from build123d import *

# Parameters (mm, degrees)
SKETCH006_W     = 266
SKETCH006_H     = 48
PAD003_DEPTH    = 4
SKETCH024_W     = 40
SKETCH024_H     = 30
SKETCH024_W_2   = 30
SKETCH024_H_2   = 20
POCKET007_DEPTH = 4.001
SKETCH031_R     = 12
SKETCH031_R_2   = 1.6
POCKET014_DEPTH = 4.001
SKETCH040_R     = 1.65
HOLE005_DEPTH   = 4.001
SKETCH055_W     = 76
SKETCH055_H     = 10
POCKET021_DEPTH = 4.001


with BuildPart() as part:
    # Sketch006 (on DatumPlane) → Pad003 (new body)
    with BuildSketch(Plane.XZ.offset(-79)):
        with Locations((0, 16)):
            Rectangle(SKETCH006_W, SKETCH006_H)
    extrude(amount=PAD003_DEPTH)

    # Sketch024 (on Face5 of Pad003) → Pocket007 (cut, through all)
    with BuildSketch(Plane(origin=(0, 79, 0), x_dir=(1, 0, 0), z_dir=(0, 1, 0))):
        Polygon((-145, 30), (-100, 30), (-100, 0), (-125, 0), (-125, -15.5), (-155, -15.5), (-155, 4.5), (-145, 4.5), align=None)
        with Locations((-40, 15)):
            Rectangle(SKETCH024_W, SKETCH024_H)
        with Locations((40, 15)):
            Rectangle(SKETCH024_W, SKETCH024_H)
        Polygon((100, 30), (145, 30), (145, 4.5), (155, 4.5), (155, -15.5), (125, -15.5), (125, 0), (100, 0), align=None)
        with Locations((-140, -37.5)):
            Rectangle(SKETCH024_W_2, SKETCH024_H_2)
        with Locations((140, -37.5)):
            Rectangle(SKETCH024_W_2, SKETCH024_H_2)
    extrude(amount=-POCKET007_DEPTH, mode=Mode.SUBTRACT)

    # Sketch031 (on Face2 of Pocket007) → Pocket014 (cut, through all)
    with BuildSketch(Plane(origin=(0, 79, 0), x_dir=(1, 0, 0), z_dir=(0, 1, 0))):
        with Locations((-107, -20.5)):
            Circle(SKETCH031_R)
        with Locations((-116.5, -8.5)):
            Circle(SKETCH031_R_2)
        with Locations((-97.5, -32.5)):
            Circle(SKETCH031_R_2)
        with Locations((-88.5, -8.5)):
            Circle(SKETCH031_R_2)
        with Locations((-79, -20.5)):
            Circle(SKETCH031_R)
        with Locations((-69.5, -32.5)):
            Circle(SKETCH031_R_2)
    extrude(amount=-POCKET014_DEPTH, mode=Mode.SUBTRACT)

    # Sketch040 (on Face2 of Pocket014) → Hole005 (cut, through all)
    with BuildSketch(Plane(origin=(0, 79, 0), x_dir=(1, 0, 0), z_dir=(0, 1, 0))):
        with Locations((39.5, -27)):
            Circle(SKETCH040_R)
    extrude(amount=-HOLE005_DEPTH, mode=Mode.SUBTRACT)

    # Sketch055 (on Face2 of Pocket007) → Pocket021 (cut, through all)
    with BuildSketch(Plane(origin=(0, 79, 0), x_dir=(1, 0, 0), z_dir=(0, 1, 0))):
        with Locations((-91, -41)):
            Rectangle(SKETCH055_W, SKETCH055_H)
    extrude(amount=-POCKET021_DEPTH, mode=Mode.SUBTRACT)


solid = part.part
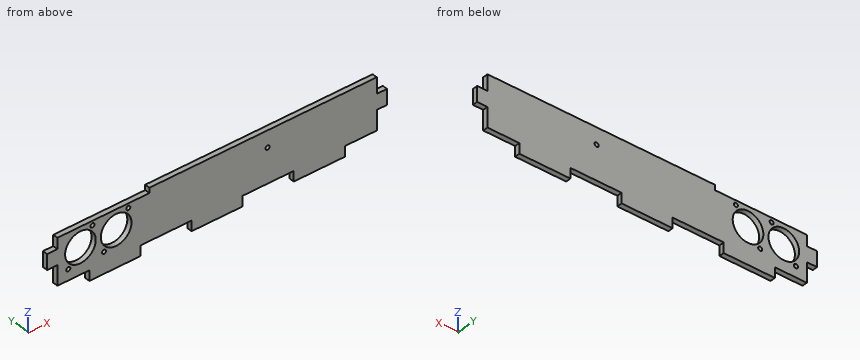
Geometry check sheet. Reference: the model listing, model coordinates, mm. Give positions to 0.01 mm unless a question says otherwise; leave off trailing zeros. Order: outer loops, then holes, each group sorted by start corner. A loop starts at its lowest first (then second) coordinate and runs counter-clockwise, first axis right, second up. Notation, with made-up numbers: (19, 0.5) - (56, 0.5) arc R10 ccw to (56, 4.5) - close; hole circle Ø6 at (-39, -37). An arc over 180 degrees is marked (long way). Answer as a JSON object with one key per item and string values.
(1) Material ranges on line 1 (X direction, y = 77.8, z = -6); line 2 (X direction, y = 76.25, z = 27); line 3 (Z direction, x = -107, y = 77.95), recorded low to high.
Report:
{"line 1": "-100 to -60, -20 to 20, 60 to 100", "line 2": "-133 to -117.09, -96.91 to -89.09, -68.91 to 37.85, 41.15 to 133", "line 3": "0 to 8.5, 32.5 to 36"}
(2) Cross-section at B-B (x = -107). Record the cut outline in (y, z).
Report:
{"outline": "(75, 0) - (79, 0) - (79, 8.5) - (75, 8.5) - close; (75, 32.5) - (79, 32.5) - (79, 36) - (75, 36) - close"}
(3) Depth check by flat-ended pin: pin 1 Ø1.2 at (y, z) = (76.5, -2) entering from +X; pin 2 Ø1.2 at (y, z) = (78, -4.5) entering from -X; pin 3 Ø3.5 at (x, z) = (-88.5, 8.5) entering from +Y; pin 4 Ø1.2 at (x, y) = (38, 76) entering from -Z. Enter the tip coordinate at first touch or a pass-through.
Report:
{"pin 1": "x = 100", "pin 2": "x = -100", "pin 3": "y = 79", "pin 4": "z = 0"}
(4) Cross-section at C-C (y = 76.65). State how many separate pieces and enclosed holes the cut face has, then the cut area to 3 significant figures.
Report:
{"separate pieces": "1", "enclosed holes": "7", "area": "9,920 mm^2"}
(5) Cross-section at D-D (z = -2.5). Record the cut outline in (x, y), then the cut area to 3 significant figures.
Report:
{"outline": "(-100, 75) - (-60, 75) - (-60, 79) - (-100, 79) - close; (-20, 75) - (20, 75) - (20, 79) - (-20, 79) - close; (60, 75) - (100, 75) - (100, 79) - (60, 79) - close", "area": "480 mm^2"}
(6) Cross-section at A-A (z = 20.5). Record the cut outline in (x, y), then the cut area to 3 significant figures.
Report:
{"outline": "(-133, 75) - (-119, 75) - (-119, 79) - (-133, 79) - close; (-95, 75) - (-91, 75) - (-91, 79) - (-95, 79) - close; (-67, 75) - (133, 75) - (133, 79) - (-67, 79) - close", "area": "872 mm^2"}
